Autodesk Inventor part; units mm, degrees
ref_plane "Work Plane1" through (0, 206.1678, -11.4428) normal (0, 0, -1) x (-1, 0, 0)
ref_plane "YZ Plane" through (0, 0, 0) normal (1, 0, 0) x (0, 1, 0)
ref_plane "XZ Plane" through (0, 0, 0) normal (0, 1, 0) x (-1, 0, 0)
sketch "Sketch1" plane through (0, 0, 0) normal (0, 1, 0) x (-1, 0, 0)
  circle A0 centre (0, 0) radius 0.25
  dimension "d0" = 0.5
sketch "Sketch2" plane through (0, 0, 0) normal (1, 0, 0) x (0, 1, 0)
  line L0 (0, 0) -> (66.843, 0)
  line L1 (66.843, 0) -> (131.0178, -11.4428)
  line L2 (131.0178, -11.4428) -> (206.1678, -11.4428)
  dimension "d1" = 66.843
  dimension "d2" = 169.89
  dimension "d3" = 65.187
  dimension "d4" = 75.15
sweep "Sweep1" add profiles "Sketch1" path "Sketch2"
sketch "Sketch3" plane through (0, 206.1678, -11.4428) normal (0, 1, 0) x (1, 0, 0)
  line L0 (0, 0) -> (-0.3702, 0) construction
  point P0 (0, -11.4428)
ref_plane "Work Plane1" through (0, 206.1678, -11.4428) normal (0, 0, -1) x (-1, 0, 0)
sketch "Sketch4" plane through (0, 206.1678, -11.4428) normal (0, 0, -1) x (-1, 0, 0)
  line L0 (0.25, 0) -> (-0.25, 0)
  circle A0 centre (0, 0) radius 1.5
  line L1 (0, 1.5) -> (0, 0)
  line L2 (0, 0) -> (-1.5, 0)
  point P0 (0, -206.1678)
  dimension "d8" = 3
revolve "Revolution1" add sketch "Sketch4" angle 360 about axis through (0, 207.6678, -11.4428) along (0, -1, 0) picked at (-0.1113, 0.9875) contours L0 L2 A0 L1
fillet "Fillet1" radius 0.2 1 edges at (-1.5, 206.1678, -11.4428)
sketch "Sketch5" plane through (0, 0, 0) normal (0, -1, 0) x (1, 0, 0)
  circle A0 centre (0, 0) radius 0.25
extrude "Extrusion1" add sketch "Sketch5" along normal blind 0.1
properties part number "cable anular"
Source: CAD feature listing. Evaluate the final solid. Frame: model axes, mm. Coordinates: 2 decimals unless noted, no trailing zeros. Order: outer loops, then holes, each group sorted by start corner. A loop starts at its lowest first (then second) coordinate and runs counter-clockwise, first axis right, second up.
Item 1: Material intervals for line 1 (Z direction, x = -0.15, y = 182); line 2 (Y direction, x = -0.3, z = -10.5); line 3 (Z direction, x = -0.15, y = 125), sorted ascending.
Output values:
line 1: z = -11.64 to -11.24
line 2: y = 206.17 to 207.3
line 3: z = -10.57 to -10.17
Item 2: Cut plane A-A (y = 34.5). Return loops of the section in (x, z), plus the area to 3 significant figures.
Output values:
outline: circle Ø0.5 at (0, 0)
area: 0.196 mm2
Item 3: First-contact query: P1, Ø2, axis at y = 79, z = -1.5, coming from the -X side. Flat tip, straight axial feed; report the tip coordinate or a pass-through.
Output values:
P1: stops at x = -0.25
